from build123d import *

# Parameters (mm, degrees)
F1_DEPTH = 2


with BuildPart() as f1:
    # F0 (on Top) → F1 (new body)
    with BuildSketch(Plane.XY):
        Polygon((-180, -3.5), (-180, -103.5), (-5, -103.5), (0, -103.5), (0, -98.5), (-5, -98.5), (-5, -93.5), (0, -93.5), (0, -88.5), (-5, -88.5), (-5, -83.5), (0, -83.5), (0, -78.5), (-5, -78.5), (-5, -73.5), (0, -73.5), (0, -68.5), (-5, -68.5), (-5, -63.5), (0, -63.5), (0, -58.5), (-5, -58.5), (-5, -53.5), (0, -53.5), (0, -48.5), (-5, -48.5), (-5, -43.5), (0, -43.5), (0, -38.5), (-5, -38.5), (-5, -33.5), (0, -33.5), (0, -28.5), (-5, -28.5), (-5, -23.5), (0, -23.5), (0, -18.5), (-5, -18.5), (-5, -13.5), (0, -13.5), (0, -8.5), (-5, -8.5), (-5, -3.5), (-10, -3.5), (-10, 1.5), (-15, 1.5), (-15, -3.5), (-20, -3.5), (-20, 1.5), (-25, 1.5), (-25, -3.5), (-30, -3.5), (-30, 1.5), (-35, 1.5), (-35, -3.5), (-40, -3.5), (-40, 1.5), (-45, 1.5), (-45, -3.5), (-50, -3.5), (-50, 1.5), (-55, 1.5), (-55, -3.5), (-60, -3.5), (-60, 1.5), (-65, 1.5), (-65, -3.5), (-70, -3.5), (-70, 1.5), (-75, 1.5), (-75, -3.5), (-80, -3.5), (-80, 1.5), (-85, 1.5), (-85, -3.5), (-90, -3.5), (-90, 1.5), (-95, 1.5), (-95, -3.5), (-100, -3.5), (-100, 1.5), (-105, 1.5), (-105, -3.5), (-110, -3.5), (-110, 1.5), (-115, 1.5), (-115, -3.5), (-120, -3.5), (-120, 1.5), (-125, 1.5), (-125, -3.5), (-130, -3.5), (-130, 1.5), (-135, 1.5), (-135, -3.5), (-140, -3.5), (-140, 1.5), (-145, 1.5), (-145, -3.5), (-150, -3.5), (-150, 1.5), (-155, 1.5), (-155, -3.5), (-160, -3.5), (-160, 1.5), (-165, 1.5), (-165, -3.5), (-170, -3.5), (-170, 1.5), (-175, 1.5), (-175, -3.5), align=None)
    extrude(amount=F1_DEPTH)


solid = f1.part
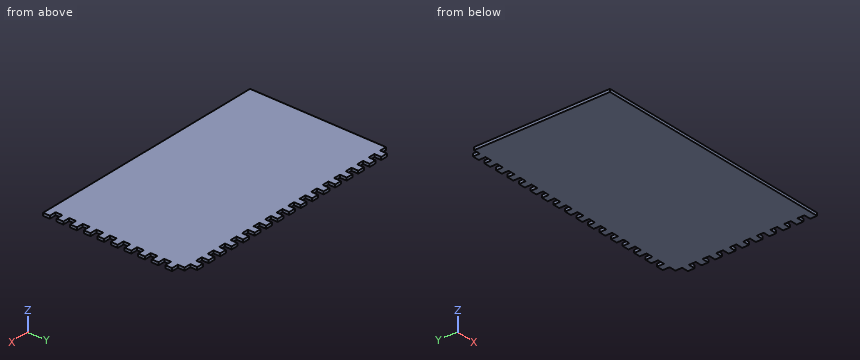
Check sheet for the modelled part. Datum: model origin and axes. Units: mm. Round coordinates to 2 decimals unless told otherwise and drop trailing zeros. Loops run counter-clockwise (first coordinate to the right, second up) from the corner with the lowest first, then second, coordinate; pieces in that order, holes last. Notation, with made-up numbers: M 18.5,2.5 L 36.5,2.5 A11 ccw 36.5,10.5 Z; hole C 25.25,33 d10. An arc over 180 degrees is marked long. One line per item, written item: value.
(1) Sectioned sample at B-B, the plane y = -66. Record the cut outline in (x, z), then the cut area to 3 significant figures.
Computed values:
outline: M -180,0 L -5,0 L -5,2 L -180,2 Z
area: 350 mm^2
(2) Sectioned sample at A-A, the plane x = -28. Record the cut outline in (y, z), then the cut area to 3 significant figures.
Computed values:
outline: M -103.5,0 L -3.5,0 L -3.5,2 L -103.5,2 Z
area: 200 mm^2
(3) Thickness scan on line 1 (X direction, y = -17, z = 1.8); line 2 (Y direction, x = -138.5, z = 0.8). Record the ranges inside material, lowest first.
Computed values:
line 1: x = -180 to -5
line 2: y = -103.5 to -3.5
(4) Depth check by flat-ended pin: pin 1 Ø0.6 at (y, z) = (-96, 1.5) entering from +X; pin 2 Ø0.6 at (x, z) = (-28.5, 1) entering from +Y; pin 3 Ø5 at (x, y) = (-83, -33) entering from -Z; pin 4 Ø1 at (y, z) = (-0.5, 1) entering from -X. Enter the tip coordinate at first touch or a pass-through.
Computed values:
pin 1: stops at x = -5
pin 2: stops at y = -3.5
pin 3: stops at z = 0
pin 4: stops at x = -175
